Read the model definition and answer for the solid it produces. Units are mm, in the model's axes. A direction names the side the tool comes from. Coordinates: 2 decimals unless noted, no trailing zeros. Write each loop counter-clockwise with the first axis right and the second up, starting at its lowest first coordinate (ties: lowest second). Pieces come first, ordered by that corner, then holes. Notation, with made-up numbers: M 3,50 L 10,50 A18 ccw 10,83 Z; hole C -29.75,-0.75 d4. An arc over 180 degrees is marked long. Write item = value, one per line.
Autodesk Inventor part; units mm, degrees
ref_plane "Work Plane1" through (29, 0, 0) normal (0, -1, 0) x (1, 0, 0)
ref_plane "YZ Plane" through (0, 0, 0) normal (1, 0, 0) x (0, 1, 0)
ref_plane "XZ Plane" through (0, 0, 0) normal (0, 1, 0) x (-1, 0, 0)
sketch "Sketch1" plane through (0, 0, 0) normal (0, 0, 1) x (1, 0, 0)
  line L0 (-0.9667, 0) -> (25, 0)
  line L1 (25, 0) -> (25, 2.5)
  line L2 (25, 2.5) -> (9, 2.5)
  line L3 (9, 2.5) -> (8.5091, 2.5)
  line L4 (8.5091, 2.5) -> (0, 2.5)
  line L5 (0, 2.5) -> (0, 4.25)
  line L6 (0, 4.25) -> (-5, 4.25)
  line L7 (-5, 4.25) -> (-5, 2.3094)
  line L8 (-5, 2.3094) -> (-2.3, 2.3094)
  line L9 (-2.3, 2.3094) -> (-0.9667, 0)
  line L10 (-11, 0) -> (31, 0)
  line L11 (0, -0.85) -> (0, 5.1)
  line L12 (9, 2.5) -> (0, 2.5) construction
  dimension "d1" = 16
  dimension "d2" = 0.4909
  dimension "d3" = 5
  dimension "d4" = 2.7
  dimension "d5" = 60
  dimension "d6" = 5
  dimension "d7" = 5
  dimension "d8" = 4.6188
  dimension "d9" = 8.5
  dimension "d26" = 25
revolve "Body" add sketch "Sketch1" angle 360 about axis through (-0.9667, 0, 0) along (1, 0, 0)
sketch "Sketch2" plane through (-5, 0, 0) normal (-1, 0, 0) x (0, 0, 1)
  circle A0 centre (0, 0) radius 2.3094
  line L0 (0, -5.95) -> (0, 5.95)
  line L1 (-5.95, 0) -> (5.95, 0)
  line L2 (2.3094, 0) -> (1.1547, -2)
  line L3 (1.1547, -2) -> (-1.1547, -2)
  line L4 (-1.1547, -2) -> (-2.3094, 0)
  line L5 (-2.3094, 0) -> (-1.1547, 2)
  line L6 (-1.1547, 2) -> (1.1547, 2)
  line L7 (1.1547, 2) -> (2.3094, 0)
extrude "Slot" add sketch "Sketch2" against normal up to next contours L7 A0 | A0 L2 | L6 L0 A0 | A0 L0 L3 | L0 L6 A0 | A0 L3 L0 | L4 A0 | A0 L5
fillet "Fillet1" radius 0.4 1 edges at (-5, -4.25, 0)
thread "Thread"
chamfer "Chamfer1" distance 0.4908 distance2 0.4908 1 edges at (25, -2.5, 0) measured on face at (25, 0.6587, -0.3326)
ref_plane "Work Plane1" through (29, 0, 0) normal (0, -1, 0) x (1, 0, 0)
fillet "Fillet2" radius 0.1 1 edges at (0, -2.5, 0)
equation "\"d30\" = R"
equation "\"d17\" = RR"
equation "\"d13\" = GEL"
equation "\"d15\" = -0.5 * SPD + 0.5 * GD"
equation "\"d16\" = GUL"
equation "\"d1\" = GEL"
equation "\"d3\" = KOH"
equation "\"d4\" = INTI"
equation "\"d6\" = GD"
equation "\"d7\" = BDM"
equation "\"d8\" = 1.1547 * SW"
equation "\"d9\" = KOD"
equation "\"d26\" = NLG"
equation "\"GD\" = NND"
equation "\"NLG\" = 25"
equation "\"GEL\" = 16"
equation "\"KOD\" = 8.5"
equation "\"KOH\" = NND"
equation "\"INTI\" = 2.7"
equation "\"GAL\" = 0.61345 * PTC"
equation "\"GUL\" = 0.61345 * PTC"
equation "\"BDM\" = NND"
equation "\"SW\" = 4"
equation "\"RR\" = 0.4"
equation "\"SPD\" = NND - 1.2269 * PTC"
equation "\"R\" = 0.1"
equation "\"TOA\" = 30deg"
equation "\"GD1\" = THREADDIA - 1.2269 * PTC"
equation "\"THREADDIA\" = 5"
equation "\"FAWI\" = 45deg"
equation "\"PTC\" = 0.8"
equation "\"NND\" = 5"
equation "\"E0\" = 1.155 * SW"
equation "\"PHH\" = 0"
properties part number "CSN 02 1143 - M5 x 25" material "Steel, Mild"
Item 1: Flat-ended cylindrical pins translate along their axes: pin 1 (2 mm diameter, centred on x = 2, y = -3, fed in from +Z); pin 2 (1 mm diameter, centred on x = 19.5, z = -2.5, fed in from +Y); pin 3 (3 mm diameter, centred on x = 12, z = 0, fed in from +Y). Find the tip coordinate at first contact, or state that the pin passes through.
Worked answers:
pin_1 = 1.5
pin_2 = 1.5
pin_3 = 2.5
Item 2: For a pull along Z with two mould halves and no side action, classify faces 1 (the face through (-3.581, 1.014, 1.724)), 2 (the face through (-2.332, 2.285, -3.584)), 3 (the face through (25, 0, 0)) as released by +Z, released by -Z, zero draft, split by the parting line, or undercut.
Worked answers:
face_1 = undercut
face_2 = split by the parting line
face_3 = zero draft
Item 3: Consider line 1 along X through (y, z) = (2.5, 1.75); line 2 along Z through (x, y) = (21.5, 1.5). Determine where each line is inside the solid, lowest interval first. Write a range as from..to.
Worked answers:
line_1 = -5..0
line_2 = -2..2
Item 4: Find section A-A (x = -3). Determine the outline of the cut face in (y, z), and give its area (3 significant figures).
Worked answers:
outline = C 0,0 d8.5; hole M -2,-1.15 L 0,-2.31 L 2,-1.15 L 2,1.15 L 0,2.31 L -2,1.15 Z
area = 42.9 mm²
Item 5: Find section B-B (x = 8). Determine the outline of the cut face in (y, z).
Worked answers:
outline = C 0,0 d5
Item 6: Which of the six approach directions +Z, -Z, +X, -X, +Y, -Y give full straight-line access (tool end or side, diameter ignored) to faces 4 (the face through (-5, -2, 2)), 5 (the face through (0, 2, 2)), 6 (the face through (-3.581, -1.014, -1.724))?
Worked answers:
face_4 = +Z, -Z, -X, +Y, -Y
face_5 = +X
face_6 = -X
